from build123d import *

# Parameters (mm, degrees)
SKETCH1_W           = 122
SKETCH1_H           = 90
BOSS_EXTRUDE1_DEPTH = 3
SKETCH2_W           = 10
SKETCH2_H           = 10
BOSS_EXTRUDE2_DEPTH = 6
CUT_EXTRUDE2_REACH  = 153.872
SKETCH4_R           = 1.5
CUT_EXTRUDE3_REACH  = 153.872
SKETCH5_R           = 1.5
SKETCH7_W           = 6
SKETCH7_H           = 3
SKETCH7_W_2         = 3
SKETCH7_H_2         = 6
SKETCH7_W_3         = 21
SKETCH7_H_3         = 55
CUT_EXTRUDE4_DEPTH  = 152.7234326


with BuildPart() as part:
    # Sketch1 → Boss-Extrude1 (new body)
    with BuildSketch(Plane(origin=(0, 0, 0), x_dir=(1, 0, 0), z_dir=(0, 1, 0))):
        with Locations((61, 45)):
            Rectangle(SKETCH1_W, SKETCH1_H)
    extrude(amount=BOSS_EXTRUDE1_DEPTH)

    # Sketch2 → Boss-Extrude2 (add)
    with BuildSketch(Plane(origin=(0, 3, 0), x_dir=(1, 0, 0), z_dir=(0, 1, 0))):
        Polygon((0, 0), (10, 0), (10, 5.706645394), (10, 10), (7.781127404, 10), (0, 10), align=None)
        with Locations((5, 85)):
            Rectangle(SKETCH2_W, SKETCH2_H)
        with Locations((117, 85)):
            Rectangle(SKETCH2_W, SKETCH2_H)
        with Locations((117, 5)):
            Rectangle(SKETCH2_W, SKETCH2_H)
    extrude(amount=BOSS_EXTRUDE2_DEPTH)

    # Sketch4 → Cut-Extrude2 (cut, up to next)
    with BuildSketch(Plane.ZY, mode=Mode.PRIVATE) as cut_extrude2_sk1:
        with Locations((-85, 4.5)):
            Circle(SKETCH4_R)
    cut_extrude2_tool1 = extrude(cut_extrude2_sk1.sketch, amount=-CUT_EXTRUDE2_REACH, mode=Mode.PRIVATE) & part.part
    # Sketch4 → Cut-Extrude2 (cut, up to next)
    with BuildSketch(Plane.ZY, mode=Mode.PRIVATE) as cut_extrude2_sk2:
        with Locations((-5, 4.5)):
            Circle(SKETCH4_R)
    cut_extrude2_tool2 = extrude(cut_extrude2_sk2.sketch, amount=-CUT_EXTRUDE2_REACH, mode=Mode.PRIVATE) & part.part
    add(cut_extrude2_tool1.solids().sort_by_distance((0, 4.5, -85))[0], mode=Mode.SUBTRACT)
    add(cut_extrude2_tool2.solids().sort_by_distance((0, 4.5, -5))[0], mode=Mode.SUBTRACT)

    # Sketch5 → Cut-Extrude3 (cut, up to next)
    with BuildSketch(Plane(origin=(122, 0, 0), x_dir=(0, 0, -1), z_dir=(1, 0, 0)), mode=Mode.PRIVATE) as cut_extrude3_sk1:
        with Locations(Location((85, 4.5, 0), (0, 0, 180))):
            Circle(SKETCH5_R)
    cut_extrude3_tool1 = extrude(cut_extrude3_sk1.sketch, amount=-CUT_EXTRUDE3_REACH, mode=Mode.PRIVATE) & part.part
    # Sketch5 → Cut-Extrude3 (cut, up to next)
    with BuildSketch(Plane(origin=(122, 0, 0), x_dir=(0, 0, -1), z_dir=(1, 0, 0)), mode=Mode.PRIVATE) as cut_extrude3_sk2:
        with Locations(Location((5, 4.5, 0), (0, 0, 180))):
            Circle(SKETCH5_R)
    cut_extrude3_tool2 = extrude(cut_extrude3_sk2.sketch, amount=-CUT_EXTRUDE3_REACH, mode=Mode.PRIVATE) & part.part
    add(cut_extrude3_tool1.solids().sort_by_distance((122, 4.5, -85))[0], mode=Mode.SUBTRACT)
    add(cut_extrude3_tool2.solids().sort_by_distance((122, 4.5, -5))[0], mode=Mode.SUBTRACT)

    # Sketch7 → Cut-Extrude4 (cut, through all)
    with BuildSketch(Plane(origin=(0, 3, 0), x_dir=(1, 0, 0), z_dir=(0, 1, 0))):
        with Locations((48, 74.815523004)):
            Rectangle(SKETCH7_W, SKETCH7_H)
        with Locations((114, 75.116921084)):
            Rectangle(SKETCH7_W, SKETCH7_H)
        with Locations((48, 11.815523004)):
            Rectangle(SKETCH7_W, SKETCH7_H)
        with Locations((114, 12.116921084)):
            Rectangle(SKETCH7_W, SKETCH7_H)
        with Locations((110.5, 82.616921084)):
            Rectangle(SKETCH7_W_2, SKETCH7_H_2)
        with Locations((103.5, 82.616921084)):
            Rectangle(SKETCH7_W_2, SKETCH7_H_2)
        with Locations((10.5, 41.5)):
            Rectangle(SKETCH7_W_3, SKETCH7_H_3)
    extrude(amount=-CUT_EXTRUDE4_DEPTH, mode=Mode.SUBTRACT)


solid = part.part
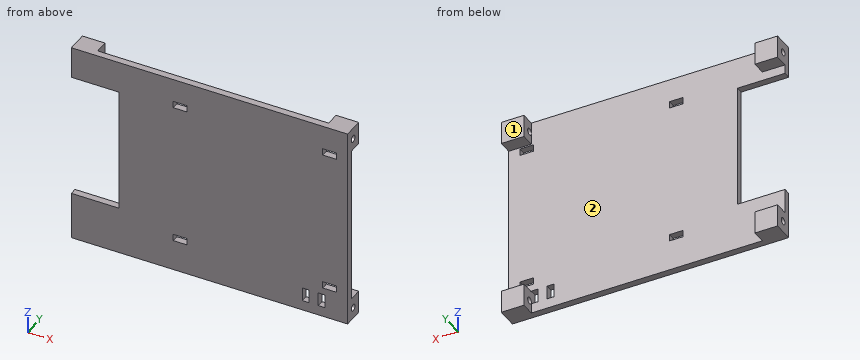
Source: CAD feature listing. Evaluate the final solid. Frame: model axes, mm. Face numbers are marked on the shaded views. Round coordinates to 2 decimals unless told otherwise and drop trailing zeros. Loops run counter-clockwise (first coordinate to the right, second up) from the corner with the lowest first, then second, coordinate; pieces in that order, holes last.
Q1. Section B-B, the plane z = -51.5. Return loops of the section in (x, y).
Q2. Mould query, pull axis X, two halves, no side actions, for the marked faces 1 and 2. Classes: pulls with the +X half, pulls with the -X half, needs draft (parallel to the pull), parting line crosses it, or undercut.
Q3. Section C-C, the plane x = 29. Return loops of the section in (y, z), plus the area to 3 significant figures.
Q4. Section A-A, the plane y = 4.5. State how many separate pieces and enclosed holes the cut face has, plus the area to 3 significant figures.
Q5. Ray query, line 1 (Z direction, x = 7.5, y = 4.5); line 2 (X direction, y = 1.75, z = -81); line 3 (Y direction, x = 7.5, z = -5). Return the intervals inside material, ascending.
Q6. First-contact query: P1, Ø5, axis at y = 6.5, z = -21, coming from the +X side; P2, Ø2.5, axis at y = 1.5, z = -38, coming from the -X side. Flat tips, straight axial feed; report the tip coordinate or a pass-through.
Solutions:
1. outline: (21, 0) - (122, 0) - (122, 3) - (21, 3) - close
2. face 1: needs draft
2. face 2: undercut
3. outline: (0, -90) - (3, -90) - (3, 0) - (0, 0) - close
3. area: 270 mm2
4. separate pieces: 8
4. enclosed holes: 0
4. area: 280 mm2
5. line 1: z = -90 to -86.5, -83.5 to -80, -10 to -6.5, -3.5 to 0
5. line 2: x = 0 to 102, 105 to 109, 112 to 122
5. line 3: y = 0 to 3, 6 to 9
6. P1: passes through
6. P2: stops at x = 21
